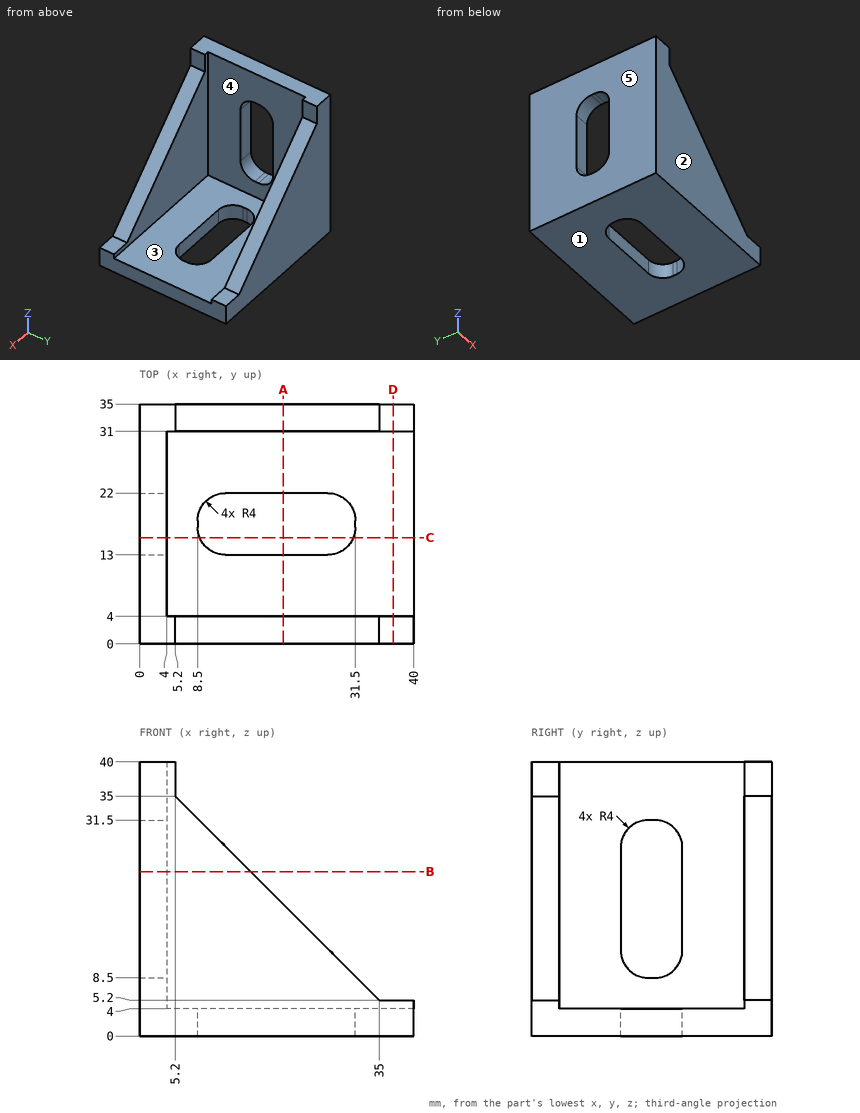
For this review, use the dimensioned drawing (mm, ordinates from the lowest corner) and the shaded views. A direction names the side the tool comes from. Give positions to 0.01 mm unless a question says otherwise; leave off trailing zeros. Order: outer loops, then holes, each group sorted by start corner. A loop starts at its lowest first (then second) coordinate and runs counter-clockwise, first axis right, second up. Notation, with made-up numbers: (85.5, -12.5) - (101.5, -12.5) arc R27 cw to (101.5, 11.5) - close; hole circle Ø8 at (69, -8). An arc over 180 degrees is marked (long way). Use CSV: the item, a comma, the result in double quotes. Start each with the question number.
Q1. Take a section at C-C (y = 15.5). State the section outline as (x, z) points, and give its area (3 significant figures).
Q2. For line 1 (Y direction, x = 15.5, z = 9); line 2 (X direction, y = 27, z = 23), list the stretches that pass through material, from the lowest coordinate up.
Q3. Take a section at A-A (x = 21). State the section outline as (y, z) points, and give its area (3 significant figures).
Q4. For P1, Ø1.2, axis at x = 38.5, y = 34, coming from the +Z side; P2, Ø2, axis at y = 33.5, z = 37, coming from the +X side; P3, Ø13.5, axis at x = 17.5, y = 14.5, coming from the +Z side, all flat-tipped, find the tip position at first contact; note any pin that passes through.
Q5. Take a section at D-D (x = 37). State the section outline as (y, z) points, and give its area (3 significant figures).
Q6. Machinability: for the marked faces 4 and 5, which of the approach directions +Z, -Z, +X, -X, +Y, -Y give a long, thin tool a straight path to every point of the face, cutting with its end or side? Answer none if there is none.
Q7. Take a section at B-B (z = 24). State the section outline as (x, y) points.
Q8. Draft analysis for pull direction Y (two halves, no side actions). For the marked faces 1, 2 and 3, state which applies: pulls with the +Y half, pulls with the -Y half, needs draft (parallel to the pull), parting line crosses it, or undercut.
Calculated:
1,outline,"(0, 0) - (8.79, 0) - (8.79, 4) - (4, 4) - (4, 8.79) - (0, 8.79) - close; (0, 31.21) - (4, 31.21) - (4, 40) - (0, 40) - close; (31.21, 0) - (40, 0) - (40, 4) - (31.21, 4) - close"
1,area,"125 mm²"
2,line 1,"y = 0 to 4, 31 to 35"
2,line 2,"x = 0 to 4"
3,outline,"(0, 0) - (13, 0) - (13, 4) - (4, 4) - (4, 19.2) - (0, 19.2) - close; (22, 0) - (35, 0) - (35, 19.2) - (31, 19.2) - (31, 4) - (22, 4) - close"
3,area,"226 mm²"
4,P1,"stops at z = 5.2"
4,P2,"stops at x = 5.2"
4,P3,"stops at z = 4"
5,outline,"(0, 0) - (35, 0) - (35, 5.2) - (31, 5.2) - (31, 4) - (4, 4) - (4, 5.2) - (0, 5.2) - close"
5,area,"150 mm²"
6,face 4,"+Z, +X"
6,face 5,"+Z, -Z, -X, +Y, -Y"
7,outline,"(0, 0) - (16.2, 0) - (16.2, 4) - (4, 4) - (4, 13) - (0, 13) - close; (0, 22) - (4, 22) - (4, 31) - (16.2, 31) - (16.2, 35) - (0, 35) - close"
8,face 1,"needs draft"
8,face 2,"pulls with the -Y half"
8,face 3,"undercut"
